Autodesk Inventor part; units mm, degrees
ref_plane "YZ Plane" through (0, 0, 0) normal (1, 0, 0) x (0, 1, 0)
ref_plane "XZ Plane" through (0, 0, 0) normal (0, 1, 0) x (-1, 0, 0)
ref_plane "XY Plane" through (0, 0, 0) normal (0, 0, 1) x (1, 0, 0)
sketch "스케치1" plane through (0, 0, 0) normal (0, 1, 0) x (-1, 0, 0)
  line L0 (-8, 28) -> (8, 28)
  line L1 (8, 28) -> (8, -28)
  line L2 (8, -28) -> (-8, -28)
  line L3 (-8, -28) -> (-8, 28)
  line L4 (-8, 28) -> (8, -28) construction
  line L5 (8, 28) -> (-8, -28) construction
  line L6 (15, -35) -> (15, 35)
  line L7 (15, 35) -> (-15, 35)
  line L8 (-15, 35) -> (-15, -35)
  line L9 (-15, -35) -> (15, -35)
  point P0 (0, 0)
  dimension "d0" = 16
  dimension "d1" = 56
  dimension "d2" = 7
extrude "돌출1" add sketch "스케치1" along normal blind 55 contours L0 L1 L2 L3 | L9 L8 L7 L6
sketch "스케치2" plane through (0, 55, 0) normal (0, 1, 0) x (1, 0, 0)
  line L0 (-15, 35) -> (-15, -35)
  line L1 (-15, -35) -> (15, -35)
  line L2 (-15, -35) -> (15, -35)
  line L3 (15, -35) -> (15, 35)
  line L4 (15, 35) -> (-15, 35)
  line L5 (-15, 35) -> (-15, -35)
  line L6 (8, 28) -> (8, -28)
  line L7 (8, -28) -> (-8, -28)
  line L8 (-8, -28) -> (-8, 28)
  line L9 (-8, 28) -> (8, 28)
  point P0 (0, 0)
  dimension "d5" = 7
extrude "돌출2" cut sketch "스케치2" against normal blind 48 contours L6 L7 L8 L9
sketch "스케치3" plane through (15, 0, 35) normal (1, 0, 0) x (0, 0, -1)
  line L0 (0, 0) -> (70, 0)
  line L1 (70, 0) -> (70, 55)
  line L2 (0, 55) -> (70, 55)
  line L3 (0, 0) -> (0, 55)
  line L4 (63, 48) -> (63, 17)
  line L5 (7, 17) -> (7, 48)
  line L6 (7, 48) -> (63, 48)
  line L7 (7, 17) -> (63, 17)
  point P0 (35, 0)
  point P1 (0, 27.5)
  dimension "d8" = 7
  dimension "d10" = 17
  dimension "d11" = 7
  dimension "d12" = 7
  dimension "d13" = 31
extrude "돌출3" cut sketch "스케치3" against normal blind 40 contours L4 L7 L5 L6
sketch "스케치4" plane through (0, 7, 0) normal (0, 1, 0) x (1, 0, 0)
  line L0 (8, -28) -> (-8, -28)
  line L1 (-8, -28) -> (-8, 28)
  line L2 (8, 28) -> (8, -28)
  line L3 (8, -28) -> (-8, -28)
  line L4 (8, -21) -> (-8, -21)
  point P0 (0, 0)
  dimension "d16" = 7
extrude "돌출4" cut sketch "스케치4" against normal blind 10
sketch "스케치6" plane through (-15, 0, -35) normal (-1, 0, 0) x (0, 0, 1)
  line L0 (0, 0) -> (70, 0)
  line L1 (35, 0) -> (35, 55)
  line L2 (7, 55) -> (63, 55)
  line L3 (23, 12) -> (47, 12)
  line L4 (47, 0) -> (47, 12)
  line L5 (23, 0) -> (23, 12)
  dimension "d20" = 12
  dimension "d21" = 12
  dimension "d22" = 12
extrude "돌출5" add sketch "스케치6" along normal blind 70
sketch "스케치7" plane through (-15, 12, 12) normal (0, 1, 0) x (1, 0, 0)
  line L0 (-70, 24) -> (-70, 0)
  circle A0 centre (-70, 12) radius 35.75
  point P0 (15, 12)
  dimension "d25" = 71.5
extrude "돌출6" add sketch "스케치7" along normal mid plane 80
sketch "스케치8" plane through (-85, 52, 0) normal (0, 1, 0) x (1, 0, 0)
  circle A0 centre (0, 0) radius 35.75
  circle A1 centre (0, 0) radius 25.75
  point P0 (85, 0)
  dimension "d28" = 10
extrude "돌출7" cut sketch "스케치8" against normal blind 80 contours A1
equation "\"TransitionRadius\" = BendRadius"
properties part number "카메라 거치대"
For this review, take the finished solid that the model builds, in its own axes (mm). A direction names the side the tool comes from. Give positions to 0.01 mm unless a question says otherwise; leave off trailing zeros. Loops run counter-clockwise (first coordinate to the right, second up) from the corner with the lowest first, then second, coordinate; pieces in that order, holes last. Notation, with made-up numbers: M -3,-31 L 35,-31 A23 cw 35,-10 Z; hole C 41,-31 d8. An arc over 180 degrees is marked long. Answer as a JSON object with one key per item and string values. Group by question number.
Q1. Add section C-C on z = 0. Give the boundary of the cut face in (x, y), and give its area (3 significant figures).
Q2. Tool access review of faces 1 (the flat face through (-8, 52, 0)), 2 (the flat face through (0, 27, 35)), 3 (the flat face through (-70, 52, 23)): name each direction out of +Z, -Z, +X, -X, +Y, -Y from which nothing blocks a thin tool from reaching the whole face with its end or side.
Q3. Mouldability with a two-part tool opening along Z and no side actions: class faces 4 (the flat face through (0, 28, 28)), 5 (the flat face through (15, 15, 0)), 6 (the flat face through (0, 27, -35)), 7 (the flat face through (12, 17, 0)) as +Z half, -Z half, draft (parallel to the pull), parting line (faces both ways), or undercut.
Q4. Insertion check: P1, Ø3.5, axis at y = 51.5, z = -9.5, coming from the -X side; P2, Ø2, axis at x = -2, y = 4.5, coming from the +Z side; P3, Ø2, axis at x = -11.5, z = -12.5, coming from the -Y side. Each pin has a flat end and moves straight along its axis. Give the tip position at first contact, or say it passes through.
Q5. Add section B-B on x = -85. Give the boundary of the cut face in (y, z).
Q6. Add section A-A on y = 15.5. Give the boundary of the cut face in (x, z).
Q7. Add section D-D on y = 5.5. Give the boundary of the cut face in (x, z).
Q8. For probe 1 along Z at (x, y) = (-12, 33.5); probe 2 along X at (y, z) = (24, 0); probe 3 along Z at (x, y) = (-85, 23), list the stretches that pass through material, from the lowest coordinate up. Write a range as [from, to].
Checked values:
{
 "1": {"outline": "M -120.75,-28 L -110.75,-28 L -110.75,52 L -120.75,52 Z; M -59.25,-28 L -49.25,-28 L -49.25,0 L 15,0 L 15,17 L 8,17 L 8,7 L -8,7 L -8,17 L -15,17 L -15,12 L -49.25,12 L -49.25,52 L -59.25,52 Z; M -15,48 L -8,48 L -8,55 L -15,55 Z; M 8,48 L 15,48 L 15,55 L 8,55 Z", "area": "2,460 mm²"},
 "2": {"face 1": "+Y", "face 2": "+Z, +X, +Y, -Y", "face 3": "+Z, -Z, -X, +Y"},
 "3": {"face 4": "undercut", "face 5": "draft", "face 6": "-Z half", "face 7": "undercut"},
 "4": {"P1": "x = -119.9", "P2": "z = 35", "P3": "y = 0"},
 "5": {"outline": "M -28,-35.75 L 52,-35.75 L 52,-25.75 L -28,-25.75 Z; M -28,25.75 L 52,25.75 L 52,35.75 L -28,35.75 Z"},
 "6": {"outline": "C -85,0 d71.5; M -15,-35 L 15,-35 L 15,35 L -15,35 Z; hole C -85,0 d51.5; hole M -8,-28 L 8,-28 L 8,28 L -8,28 Z"},
 "7": {"outline": "M -51.32,-12 L -15,-12 L -15,-35 L 15,-35 L 15,35 L -15,35 L -15,12 L -51.32,12 A35.75 ccw long Z; hole C -85,0 d51.5; hole M -8,21 L 8,21 L 8,28 L -8,28 Z"},
 "8": {"probe 1": "[-35, -28], [28, 35]", "probe 2": "[-120.75, -110.75], [-59.25, -49.25]", "probe 3": "[-35.75, -25.75], [25.75, 35.75]"}
}
